CAD build for the part. Positions are in the model's coordinates, mm. A direction names the side the tool comes from. Round coordinates to 2 decimals unless told otherwise and drop trailing zeros. Order: outer loops, then holes, each group sorted by start corner. A loop starts at its lowest first (then second) coordinate and runs counter-clockwise, first axis right, second up.
```python
from build123d import *

# Parameters (mm, degrees)
SKETCH_1_R          = 20
SKETCH_1_R_2        = 6.5
SKETCH_1_R_3        = 1.6
EXTRUDE_1_DEPTH     = 5
SKETCH_2_W          = 50
SKETCH_2_H          = 15
SKETCH_2_R          = 1.6
EXTRUDE_2_DEPTH     = 5
EXTRUDE_START       = -5
EXTRUDE_4_DEPTH     = 5
CUT_EXTRUDE_START   = -3
SKETCH_5_R          = 9.5
SKETCH_5_R_2        = 3.5
SKETCH_5_R_3        = 1.6
SKETCH_5_R_4        = 6.5
CUT_EXTRUDE_1_DEPTH = 3
FILLET_1_R          = 2
CUT_EXTRUDE_2_DEPTH = 44.301270189


with BuildPart() as part:
    # Sketch 1 → Extrude 1 (new body)
    with BuildSketch(Plane(origin=(0, 0, 0), x_dir=(1, 0, 0), z_dir=(0, 1, 0))):
        with Locations(Location((0, 0, 0), (0, 0, 270))):
            Circle(SKETCH_1_R)
        with Locations(Location((0, 0, 0), (0, 0, 270))):
            Circle(SKETCH_1_R_2, mode=Mode.SUBTRACT)
        with Locations(Location((0, 9.5, 0), (0, 0, 270))):
            Circle(SKETCH_1_R_3, mode=Mode.SUBTRACT)
        with Locations(Location((8.227241336, -4.75, 0), (0, 0, 270))):
            Circle(SKETCH_1_R_3, mode=Mode.SUBTRACT)
        with Locations(Location((-8.227241336, -4.75, 0), (0, 0, 270))):
            Circle(SKETCH_1_R_3, mode=Mode.SUBTRACT)
    extrude(amount=EXTRUDE_1_DEPTH)



with BuildPart() as body_2:
    # Sketch 2 → Extrude 2 (new body)
    with BuildSketch(Plane(origin=(0, 5, 0), x_dir=(1, 0, 0), z_dir=(0, 1, 0))):
        with Locations((0, -27.5)):
            Rectangle(SKETCH_2_W, SKETCH_2_H)
        with Locations(Location((-20, -27.5, 0), (0, 0, 270))):
            Circle(SKETCH_2_R, mode=Mode.SUBTRACT)
        with Locations(Location((20, -27.5, 0), (0, 0, 270))):
            Circle(SKETCH_2_R, mode=Mode.SUBTRACT)
        with Locations(Location((0, -27.5, 0), (0, 0, 270))):
            Circle(SKETCH_2_R, mode=Mode.SUBTRACT)
    extrude(amount=-EXTRUDE_2_DEPTH)


with BuildPart() as part_1:
    add(part.part)

    add(body_2.part)  # Extrude 4 merges body 2
    # Sketch 4 → Extrude 4 (add)
    with BuildSketch(Plane(origin=(0, 5, 0), x_dir=(1, 0, 0), z_dir=(0, 1, 0)).offset(EXTRUDE_START)):
        with BuildLine():
            Line((-19.512195122, 4.390243902), (-25, -20))
            Line((-25, -20), (0, -20))
            ThreePointArc((0, -20), (-15.617376189, -12.493900951), (-19.512195122, 4.390243902))
        make_face()
        with BuildLine():
            ThreePointArc((20, 0), (14.142135624, -14.142135624), (0, -20))
            Line((0, -20), (25, -20))
            Line((25, -20), (19.512195122, 4.390243902))
            ThreePointArc((19.512195122, 4.390243902), (19.877674693, 2.208630521), (20, 0))
        make_face()
    extrude(amount=EXTRUDE_4_DEPTH)

    # Sketch 5 → Cut-Extrude 1 (cut)
    # profile 1 of 25: a face of its own
    with BuildSketch(Plane(origin=(0, 5, 0), x_dir=(1, 0, 0), z_dir=(0, 1, 0)).offset(CUT_EXTRUDE_START)):
        Circle(SKETCH_5_R)
    # profile 2 of 25: a face of its own
    with BuildSketch(Plane(origin=(0, 5, 0), x_dir=(1, 0, 0), z_dir=(0, 1, 0)).offset(CUT_EXTRUDE_START)):
        with Locations((-8.227241336, -4.75)):
            Circle(SKETCH_5_R_2)
        with Locations(Location((-8.227241336, -4.75, 0), (0, 0, 270))):
            Circle(SKETCH_5_R_3, mode=Mode.SUBTRACT)
    # profile 3 of 25: a face of its own
    with BuildSketch(Plane(origin=(0, 5, 0), x_dir=(1, 0, 0), z_dir=(0, 1, 0)).offset(CUT_EXTRUDE_START)):
        with Locations((-8.227241336, -4.75)):
            Circle(SKETCH_5_R_2)
        with Locations(Location((-8.227241336, -4.75, 0), (0, 0, 270))):
            Circle(SKETCH_5_R_3, mode=Mode.SUBTRACT)
    # profile 4 of 25: a face of its own
    with BuildSketch(Plane(origin=(0, 5, 0), x_dir=(1, 0, 0), z_dir=(0, 1, 0)).offset(CUT_EXTRUDE_START)):
        Circle(SKETCH_5_R)
        with Locations(Location((0, 0, 0), (0, 0, 270))):
            Circle(SKETCH_5_R_4, mode=Mode.SUBTRACT)
    # profile 5 of 25: a face of its own
    with BuildSketch(Plane(origin=(0, 5, 0), x_dir=(1, 0, 0), z_dir=(0, 1, 0)).offset(CUT_EXTRUDE_START)):
        with Locations((-8.227241336, -4.75)):
            Circle(SKETCH_5_R_2)
    # profile 6 of 25: a face of its own
    with BuildSketch(Plane(origin=(0, 5, 0), x_dir=(1, 0, 0), z_dir=(0, 1, 0)).offset(CUT_EXTRUDE_START)):
        with Locations((0, 9.5)):
            Circle(SKETCH_5_R_2)
    # profile 7 of 25: a face of its own
    with BuildSketch(Plane(origin=(0, 5, 0), x_dir=(1, 0, 0), z_dir=(0, 1, 0)).offset(CUT_EXTRUDE_START)):
        Circle(SKETCH_5_R)
        with Locations(Location((0, 0, 0), (0, 0, 270))):
            Circle(SKETCH_5_R_4, mode=Mode.SUBTRACT)
    # profile 8 of 25: a face of its own
    with BuildSketch(Plane(origin=(0, 5, 0), x_dir=(1, 0, 0), z_dir=(0, 1, 0)).offset(CUT_EXTRUDE_START)):
        with Locations((-8.227241336, -4.75)):
            Circle(SKETCH_5_R_2)
    # profile 9 of 25: a face of its own
    with BuildSketch(Plane(origin=(0, 5, 0), x_dir=(1, 0, 0), z_dir=(0, 1, 0)).offset(CUT_EXTRUDE_START)):
        with Locations((0, 9.5)):
            Circle(SKETCH_5_R_2)
        with Locations(Location((0, 9.5, 0), (0, 0, 270))):
            Circle(SKETCH_5_R_3, mode=Mode.SUBTRACT)
    # profile 10 of 25: a face of its own
    with BuildSketch(Plane(origin=(0, 5, 0), x_dir=(1, 0, 0), z_dir=(0, 1, 0)).offset(CUT_EXTRUDE_START)):
        Circle(SKETCH_5_R)
        with Locations(Location((0, 0, 0), (0, 0, 270))):
            Circle(SKETCH_5_R_4, mode=Mode.SUBTRACT)
    # profile 11 of 25: a face of its own
    with BuildSketch(Plane(origin=(0, 5, 0), x_dir=(1, 0, 0), z_dir=(0, 1, 0)).offset(CUT_EXTRUDE_START)):
        Circle(SKETCH_5_R)
    # profile 12 of 25: a face of its own
    with BuildSketch(Plane(origin=(0, 5, 0), x_dir=(1, 0, 0), z_dir=(0, 1, 0)).offset(CUT_EXTRUDE_START)):
        with Locations((0, 9.5)):
            Circle(SKETCH_5_R_2)
        with Locations(Location((0, 9.5, 0), (0, 0, 270))):
            Circle(SKETCH_5_R_3, mode=Mode.SUBTRACT)
    # profile 13 of 25: a face of its own
    with BuildSketch(Plane(origin=(0, 5, 0), x_dir=(1, 0, 0), z_dir=(0, 1, 0)).offset(CUT_EXTRUDE_START)):
        Circle(SKETCH_5_R)
    # profile 14 of 25: a face of its own
    with BuildSketch(Plane(origin=(0, 5, 0), x_dir=(1, 0, 0), z_dir=(0, 1, 0)).offset(CUT_EXTRUDE_START)):
        with Locations((8.227241336, -4.75)):
            Circle(SKETCH_5_R_2)
        with Locations(Location((8.227241336, -4.75, 0), (0, 0, 270))):
            Circle(SKETCH_5_R_3, mode=Mode.SUBTRACT)
    # profile 15 of 25: a face of its own
    with BuildSketch(Plane(origin=(0, 5, 0), x_dir=(1, 0, 0), z_dir=(0, 1, 0)).offset(CUT_EXTRUDE_START)):
        with Locations((8.227241336, -4.75)):
            Circle(SKETCH_5_R_2)
        with Locations(Location((8.227241336, -4.75, 0), (0, 0, 270))):
            Circle(SKETCH_5_R_3, mode=Mode.SUBTRACT)
    # profile 16 of 25: a face of its own
    with BuildSketch(Plane(origin=(0, 5, 0), x_dir=(1, 0, 0), z_dir=(0, 1, 0)).offset(CUT_EXTRUDE_START)):
        Circle(SKETCH_5_R)
        with Locations(Location((0, 0, 0), (0, 0, 270))):
            Circle(SKETCH_5_R_4, mode=Mode.SUBTRACT)
    # profile 17 of 25: a face of its own
    with BuildSketch(Plane(origin=(0, 5, 0), x_dir=(1, 0, 0), z_dir=(0, 1, 0)).offset(CUT_EXTRUDE_START)):
        with Locations((8.227241336, -4.75)):
            Circle(SKETCH_5_R_2)
    # profile 18 of 25: a face of its own
    with BuildSketch(Plane(origin=(0, 5, 0), x_dir=(1, 0, 0), z_dir=(0, 1, 0)).offset(CUT_EXTRUDE_START)):
        Circle(SKETCH_5_R)
        with Locations(Location((0, 0, 0), (0, 0, 270))):
            Circle(SKETCH_5_R_4, mode=Mode.SUBTRACT)
    # profile 19 of 25: a face of its own
    with BuildSketch(Plane(origin=(0, 5, 0), x_dir=(1, 0, 0), z_dir=(0, 1, 0)).offset(CUT_EXTRUDE_START)):
        with Locations((0, 9.5)):
            Circle(SKETCH_5_R_2)
    # profile 20 of 25: a face of its own
    with BuildSketch(Plane(origin=(0, 5, 0), x_dir=(1, 0, 0), z_dir=(0, 1, 0)).offset(CUT_EXTRUDE_START)):
        with Locations((-8.227241336, -4.75)):
            Circle(SKETCH_5_R_2)
    # profile 21 of 25: a face of its own
    with BuildSketch(Plane(origin=(0, 5, 0), x_dir=(1, 0, 0), z_dir=(0, 1, 0)).offset(CUT_EXTRUDE_START)):
        Circle(SKETCH_5_R)
        with Locations(Location((0, 0, 0), (0, 0, 270))):
            Circle(SKETCH_5_R_4, mode=Mode.SUBTRACT)
    # profile 22 of 25: a face of its own
    with BuildSketch(Plane(origin=(0, 5, 0), x_dir=(1, 0, 0), z_dir=(0, 1, 0)).offset(CUT_EXTRUDE_START)):
        with Locations(Location((0, 0, 0), (0, 0, 270))):
            Circle(SKETCH_5_R_4)
    # profile 23 of 25: a face of its own
    with BuildSketch(Plane(origin=(0, 5, 0), x_dir=(1, 0, 0), z_dir=(0, 1, 0)).offset(CUT_EXTRUDE_START)):
        with Locations((8.227241336, -4.75)):
            Circle(SKETCH_5_R_2)
    # profile 24 of 25: a face of its own
    with BuildSketch(Plane(origin=(0, 5, 0), x_dir=(1, 0, 0), z_dir=(0, 1, 0)).offset(CUT_EXTRUDE_START)):
        with Locations((8.227241336, -4.75)):
            Circle(SKETCH_5_R_2)
    # profile 25 of 25: a face of its own
    with BuildSketch(Plane(origin=(0, 5, 0), x_dir=(1, 0, 0), z_dir=(0, 1, 0)).offset(CUT_EXTRUDE_START)):
        with Locations(Location((0, 0, 0), (0, 0, 270))):
            Circle(SKETCH_5_R_4)
    extrude(amount=CUT_EXTRUDE_1_DEPTH, mode=Mode.SUBTRACT)

    # Fillet 1
    fillet_1_edges = [part_1.edges().sort_by_distance(p)[0] for p in [
        (-25, 2.5, 20),
        (25, 2.5, 20),
        (25, 2.5, 35),
        (-25, 2.5, 35),
    ]]
    fillet(fillet_1_edges, radius=FILLET_1_R)

    # Sketch 6 → Cut-Extrude 2 (cut, through all)
    with BuildSketch(Plane.XZ):
        with BuildLine():
            Line((20, 25.9), (17, 25.9))
            ThreePointArc((17, 25.9), (15.4, 27.5), (17, 29.1))
            Line((17, 29.1), (20, 29.1))
            ThreePointArc((20, 29.1), (21.6, 27.5), (20, 25.9))
        make_face()
        with BuildLine():
            Line((0, 25.9), (-3, 25.9))
            ThreePointArc((-3, 25.9), (-4.6, 27.5), (-3, 29.1))
            Line((-3, 29.1), (0, 29.1))
            ThreePointArc((0, 29.1), (1.6, 27.5), (0, 25.9))
        make_face()
        with BuildLine():
            Line((-20, 25.9), (-23, 25.9))
            ThreePointArc((-23, 25.9), (-24.6, 27.5), (-23, 29.1))
            Line((-23, 29.1), (-20, 29.1))
            ThreePointArc((-20, 29.1), (-18.4, 27.5), (-20, 25.9))
        make_face()
    extrude(amount=-CUT_EXTRUDE_2_DEPTH, mode=Mode.SUBTRACT)


solid = part_1.part
```
1. Mould opens along X. For faces 4 (the face through (-25, 3, 27)), 5 (the face through (0, 2, -20)), 6 (the face through (0, 3, -13)) say: released by +X, released by -X, zero draft, split by the parting line, or undercut.
2. Cut at A-A, the plane z = 0. Write the cut outline in (x, y), and give its area (3 significant figures).
3. Drill centre lines: line 1 (X direction, y = 2.2, z = 28); line 2 (Z direction, x = -4, y = 4.65); line 3 (Z direction, x = -2.5, y = 4.5). Where is each one in solid material? Low to high.
4. Pin check, flat tips, straight feed: P1, Ø1.5, axis at x = 18.5, y = 2, coming from the -Z side; P2, Ø5.5, axis at x = 0, z = -9.5, coming from the +Y side; P3, Ø2, axis at x = -16.5, y = 2.5, coming from the -Z side. Stop position of each tip, or through.
5. Cut at D-D, the plane y = 3.5. Write the cut outline in (x, z).
6. Cut at C-C, the plane z = 27.5. Write the cut outline in (x, y).
7. Cut at B-B, the plane x = 7.5. Write the cut outline in (y, z), and give its area (3 significant figures).
8. Tool access for faces 1 (the face through (-11.3, 3.479, 6.425)), 2 (the face through (-24.6, 2.5, 27.5)), 3 (the face through (22.27, 2.46, 7.87)): list every direction of +Z, -Z, +X, -X, +Y, -Y with a clear straight run to the whole face (end or side of a thin tool).
Outcome:
1. face 4: released by -X
1. face 5: split by the parting line
1. face 6: undercut
2. outline: (-20.5, 0) - (-6.5, 0) - (-6.5, 2) - (-9.5, 2) - (-9.5, 5) - (-20.5, 5) - close; (6.5, 0) - (20.5, 0) - (20.5, 5) - (9.5, 5) - (9.5, 2) - (6.5, 2) - close
2. area: 122 mm2
3. line 1: x = -25 to -24.52, -18.48 to -4.52, 1.52 to 15.48, 21.52 to 25
3. line 2: z = -19.6 to -8.62, 8.62 to 26.25, 28.75 to 35
3. line 3: z = -19.84 to -11.95, 9.17 to 25.9, 29.1 to 35
4. P1: stops at z = -9.22
4. P2: stops at y = 2
4. P3: stops at z = -12.64
5. outline: (-25, 20.22) arc R2 ccw to (-24.95, 19.78) - (-19.51, -4.39) arc R20 ccw to (19.51, -4.39) - (24.95, 19.78) arc R2 ccw to (25, 20.22) - (25, 33) arc R2 ccw to (23, 35) - (-23, 35) arc R2 ccw to (-25, 33) - close; hole (-23, 25.9) - (-20, 25.9) arc R1.6 ccw to (-20, 29.1) - (-23, 29.1) arc R1.6 ccw to start; hole (-9.39, 1.45) arc R9.5 ccw to (-3.44, -8.86) arc R3.5 ccw (long way) to (3.44, -8.86) arc R9.5 ccw to (9.39, 1.45) arc R3.5 ccw (long way) to (5.95, 7.41) arc R9.5 ccw to (-5.95, 7.41) arc R3.5 ccw (long way) to start; hole (-3, 25.9) - (0, 25.9) arc R1.6 ccw to (0, 29.1) - (-3, 29.1) arc R1.6 ccw to start; hole (17, 25.9) - (20, 25.9) arc R1.6 ccw to (20, 29.1) - (17, 29.1) arc R1.6 ccw to start
6. outline: (-25, 0) - (-24.6, 0) - (-24.6, 5) - (-25, 5) - close; (-18.4, 0) - (-4.6, 0) - (-4.6, 5) - (-18.4, 5) - close; (1.6, 0) - (15.4, 0) - (15.4, 5) - (1.6, 5) - close; (21.6, 0) - (25, 0) - (25, 5) - (21.6, 5) - close
7. outline: (0, -18.54) - (5, -18.54) - (5, -5.83) - (2, -5.83) - (2, 3.32) - (0, 3.32) - close; (0, 6.18) - (2, 6.18) - (2, 8.17) - (5, 8.17) - (5, 35) - (0, 35) - close
7. area: 220 mm2
8. face 1: +Y
8. face 2: +Y, -Y
8. face 3: -Z, +X, +Y, -Y
